```python
from build123d import *


with BuildPart() as part:
    # Sketch1 → Revolve1 (revolve)
    with BuildSketch(Plane.XY):
        with BuildLine():
            Line((-4.5, 15.7), (-4.5, 7.8))
            ThreePointArc((-4.5, 7.8), (-4.412132034, 7.587867966), (-4.2, 7.5))
            Line((-4.2, 7.5), (4.2, 7.5))
            ThreePointArc((4.2, 7.5), (4.412132034, 7.587867966), (4.5, 7.8))
            Line((4.5, 7.8), (4.5, 15.7))
            ThreePointArc((4.5, 15.7), (4.412132034, 15.912132034), (4.2, 16))
            Line((4.2, 16), (-4.2, 16))
            ThreePointArc((-4.2, 16), (-4.412132034, 15.912132034), (-4.5, 15.7))
        make_face()
    revolve(axis=Axis((50, 0, 0), (-1, 0, 0)))

    # Sketch2 → Cut-Revolve1 (revolve, cut)
    with BuildSketch(Plane.XY):
        Polygon((-6.3, 7.5), (-4.5, 7.5), (-4.5, 10.22), (-4.48, 10.22), (-4.48, 12.08), (-4.3, 12.08), (-4.3, 13.28), (-6.3, 13.28), align=None)
    revolve(axis=Axis((50, 0, 0), (-1, 0, 0)), mode=Mode.SUBTRACT)

    # Sketch3 → Cut-Revolve2 (revolve, cut)
    with BuildSketch(Plane.XY):
        Polygon((4.3, 13.28), (4.3, 12.08), (4.48, 12.08), (4.48, 10.22), (4.5, 10.22), (4.5, 7.5), (6.3, 7.5), (6.3, 13.28), align=None)
    revolve(axis=Axis((50, 0, 0), (-1, 0, 0)), mode=Mode.SUBTRACT)


solid = part.part
```
The listing builds one solid part. Answer for the finished solid, in the listing's coordinates (mm). Give positions to 0.01 mm unless a question says otherwise; leave off trailing zeros. Write each loop counter-clockwise with the first axis right and the second up, starting at its lowest first coordinate (ties: lowest second). Pieces come first, ordered by that corner, then holes. Notation, with made-up numbers: (52, 10.5) - (104, 10.5) arc R35 cw to (104, 45.5) - close; hole circle Ø1 at (-6.75, 10). An arc over 180 degrees is marked (long way). Use one line per item in the form item = value. Start each with the question number.
1) The mould has two halves that part along Z. Classify faces 1 (the face through (-0.06, -3.47, 15.62)), 2 (the face through (-4.3, -3, 12)), 3 (the face through (4.5, 13, -4)): pulls with the +Z half, pulls with the -Z half, needs draft (parallel to the pull), parting line crosses it, or undercut.
2) Consider line 1 along Z through (x, y) = (-4.4, 0); line 2 along Z through (x, y) = (-0.5, 0). Determine where each line is inside the solid, lowest interval first. Write a range as from..to.
3) Flat-ended cylindrical pins translate along their axes: pin 1 Ø13.5 at (y, z) = (0, 0) entering from +X; pin 2 Ø13.5 at (y, z) = (-6, -1) entering from -X; pin 3 Ø4 at (x, z) = (-1.5, 4.5) entering from -Y; pin 4 Ø4 at (x, z) = (2.5, -10.5) entering from -Y. Find the tip coordinate at first contact, or state that the pin passes through.
4) Find section A-A on x = -1. Determine the outline of the cut face in (y, z).
Geometry results:
q1.face_1 = parting line crosses it
q1.face_2 = undercut
q1.face_3 = needs draft
q2.line_1 = -15.92..-13.28, -12.08..-7.58, 7.58..12.08, 13.28..15.92
q2.line_2 = -16..-7.5, 7.5..16
q3.pin_1 = through
q3.pin_2 = -4.5
q3.pin_3 = -15.8
q3.pin_4 = -13.56
q4.outline = circle Ø32 at (0, 0); hole circle Ø15 at (0, 0)
